from build123d import *
from OCP.BRepFilletAPI import BRepFilletAPI_MakeChamfer

# Parameters (mm, degrees)
BOSS_EXTRUDE1_DEPTH = 3
CHAMFER1_SIZE       = 3
CHAMFER1_SIZE_2     = 1.853922924


with BuildPart() as part:
    # Sketch1 → Boss-Extrude1 (new body)
    with BuildSketch(Plane(origin=(0, 0, 0), x_dir=(1, 0, 0), z_dir=(0, 1, 0))):
        Polygon((86.524758425, 0), (26.737620788, 82.289935321), (-70, 50.85797696), (-70, -50.85797696), (26.737620788, -82.289935321), align=None)
    extrude(amount=BOSS_EXTRUDE1_DEPTH)

    # Chamfer1
    chamfer1_edges_1 = [part.edges().sort_by_distance(p)[0] for p in [
        (-70, 3, 0),
    ]]
    chamfer1_side_1 = [part.faces().sort_by_distance(p)[0] for p in [
        (-70, 2.962921542, 0),
    ]]
    chamfer1_edges_2 = [part.edges().sort_by_distance(p)[0] for p in [
        (-21.631189606, 3, -66.573956141),
    ]]
    chamfer1_side_2 = [part.faces().sort_by_distance(p)[0] for p in [
        (-21.631189606, 2.962921542, -66.573956141),
    ]]
    chamfer1_edges_3 = [part.edges().sort_by_distance(p)[0] for p in [
        (56.631189606, 3, -41.14496766),
    ]]
    chamfer1_side_3 = [part.faces().sort_by_distance(p)[0] for p in [
        (56.631189606, 2.962921542, -41.14496766),
    ]]
    chamfer1_edges_4 = [part.edges().sort_by_distance(p)[0] for p in [
        (56.631189606, 3, 41.14496766),
    ]]
    chamfer1_side_4 = [part.faces().sort_by_distance(p)[0] for p in [
        (56.631189606, 2.962921542, 41.14496766),
    ]]
    chamfer1_edges_5 = [part.edges().sort_by_distance(p)[0] for p in [
        (-21.631189606, 3, 66.573956141),
    ]]
    chamfer1_side_5 = [part.faces().sort_by_distance(p)[0] for p in [
        (-21.631189606, 2.962921542, 66.573956141),
    ]]
    chamfer1 = BRepFilletAPI_MakeChamfer(part.part.solid().wrapped)
    for e in chamfer1_edges_1:
        chamfer1.Add(CHAMFER1_SIZE - 0.0001, CHAMFER1_SIZE_2 - 0.0001, e.wrapped, chamfer1_side_1[0].wrapped)
    for e in chamfer1_edges_2:
        chamfer1.Add(CHAMFER1_SIZE - 0.0001, CHAMFER1_SIZE_2 - 0.0001, e.wrapped, chamfer1_side_2[0].wrapped)
    for e in chamfer1_edges_3:
        chamfer1.Add(CHAMFER1_SIZE - 0.0001, CHAMFER1_SIZE_2 - 0.0001, e.wrapped, chamfer1_side_3[0].wrapped)
    for e in chamfer1_edges_4:
        chamfer1.Add(CHAMFER1_SIZE - 0.0001, CHAMFER1_SIZE_2 - 0.0001, e.wrapped, chamfer1_side_4[0].wrapped)
    for e in chamfer1_edges_5:
        chamfer1.Add(CHAMFER1_SIZE - 0.0001, CHAMFER1_SIZE_2 - 0.0001, e.wrapped, chamfer1_side_5[0].wrapped)
    add(Compound.cast(chamfer1.Shape()), mode=Mode.REPLACE)  # a hair under: the kernel refuses the full size


solid = part.part
The model under review builds one solid part; all positions refer to its coordinate system, in mm. Round coordinates to 2 decimals unless told otherwise and drop trailing zeros. Loops run counter-clockwise (first coordinate to the right, second up) from the corner with the lowest first, then second, coordinate; pieces in that order, holes last. Notation, with made-up numbers: (20, -3.5) -> (46, -3.5) arc R32 ccw to (46, 35.5) -> close; hole circle Ø11 at (-30, 61). An arc over 180 degrees is marked (long way). Return JSON: item names as keys, results as strings.
(1) Add section B-B on y = 1.1. Write out the cut boundary in (x, z).
Solved:
{"outline": "(-69.32, -50.36) -> (26.48, -81.49) -> (85.68, 0) -> (26.48, 81.49) -> (-69.32, 50.36) -> close"}
(2) For pin 1 (1 mm diameter, centred on y = 1, z = -24, fed in from -X); pin 2 (1.5 mm diameter, centred on y = 2.5, z = 21, fed in from -X); pin 3 (1 mm diameter, centred on y = 0.5, z = 25.5, fed in from +X), all flat-tipped, find the tip position at first contact; note any pin that passes through.
Solved:
{"pin 1": "x = -69.69", "pin 2": "x = -68.92", "pin 3": "x = 68.14"}
(3) For line 1 (Y direction, x = 66, z = 26); line 2 (X direction, y = 2.7, z = -10); line 3 (Z direction, x = 50.5, y = 1.6), list the stretches that pass through material, from the lowest coordinate up.
Solved:
{"line 1": "0 to 2.14", "line 2": "-68.33 to 77.2", "line 3": "-47.9 to 47.9"}
